Check sheet for the modelled part. Datum: model origin and axes. Units: mm. A direction names the side the tool comes from. Round coordinates to 2 decimals unless told otherwise and drop trailing zeros. Write each loop counter-clockwise with the first axis right and the second up, starting at its lowest first coordinate (ties: lowest second). Pieces come first, ordered by that corner, then holes. Notation, with made-up numbers: (-23.5, -34.5) -> (6.5, -34.5) arc R28 cw to (6.5, -13.5) -> close; hole circle Ø1 at (63.25, 37.25). An arc over 180 degrees is marked (long way). Write item = value, one per line.
from build123d import *

# Parameters (mm, degrees)
F1_DEPTH = 30
F3_DEPTH = 12
F5_D     = 16


with BuildPart() as f1:
    # F0 (on Right) → F1 (new body)
    with BuildSketch(Plane.YZ):
        Polygon((-20, -22.5), (20, -22.5), (110, -22.5), (110, -10.5), (20, -10.5), (20, 22.5), (-20, 22.5), align=None)
    extrude(amount=F1_DEPTH)

    # F2 (on face) → F3 (cut)
    with BuildSketch(Plane.XY.offset(-10.5)):
        with BuildLine():
            ThreePointArc((10.5, 103), (7, 106.5), (3.5, 103))
            Line((3.5, 103), (3.5, 83))
            ThreePointArc((3.5, 83), (7, 79.5), (10.5, 83))
            Line((10.5, 83), (10.5, 103))
        make_face()
        with BuildLine():
            Line((26.5, 82.575567), (26.5, 103))
            ThreePointArc((26.5, 103), (23, 106.5), (19.5, 103))
            Line((19.5, 103), (19.5, 82.575567))
            ThreePointArc((19.5, 82.575567), (23, 79.075567), (26.5, 82.575567))
        make_face()
    extrude(amount=-F3_DEPTH, mode=Mode.SUBTRACT)

    # F5 (through all)
    with Locations(Plane.XY.offset(22.5)):
        with Locations((15, -8)):
            Hole(F5_D / 2)


solid = f1.part
(1) Access from +Z, -Z, +X, -X, +Y, -Y to the whole of each face (thin tool, end or side, straight path). Record for faces 4 (the flat face through (15, 110, -17)), 5 (the flat face through (15, 20, 6)), 6 (the flat face through (10.5, 93, -16)).
Worked answers:
face_4 = +Z, -Z, +X, -X, +Y
face_5 = +Z, +X, -X, +Y
face_6 = +Z, -Z
(2) Go/stop test with flat-tipped pins: P1, Ø12, axis at y = 91, z = -14.5, coming from the -X side; P2, Ø3, axis at x = 19.5, y = 29, coming from the +Z side; P3, Ø15, axis at x = 20.5, z = 10, coming from the +Y side. Record where each tip stops, or that it passes through.
Worked answers:
P1 = 0
P2 = -10.5
P3 = 20
(3) Sectioned sample at A-A on y = -8. Enter the section's corners in (x, z), then the cut area to 3 significant figures.
Worked answers:
outline = (0, -22.5) -> (7, -22.5) -> (7, 22.5) -> (0, 22.5) -> close; (23, -22.5) -> (30, -22.5) -> (30, 22.5) -> (23, 22.5) -> close
area = 630 mm²
(4) Sectioned sample at B-B on x = 15. Enter the section's corners in (y, z).
Worked answers:
outline = (-20, -22.5) -> (-16, -22.5) -> (-16, 22.5) -> (-20, 22.5) -> close; (0, -22.5) -> (110, -22.5) -> (110, -10.5) -> (20, -10.5) -> (20, 22.5) -> (0, 22.5) -> close
(5) Release check for a two-part mould opening along X. For faces 1 (the flat face through (30, 15, -5)), 2 (the flat face through (19.5, 93, -16)), 3 (the flat face through (0, 15, -5)) record: pulls with the +X half, pulls with the -X half, needs draft (parallel to the pull), parting line crosses it, or undercut.
Worked answers:
face_1 = pulls with the +X half
face_2 = undercut
face_3 = pulls with the -X half
(6) Material ranges on L1, parallel to X at y = 86, z = -20; L2, parallel to Y at x = 15, z = -7.5; L3, parallel to Z at x = 2, y = 104, recorded low to high. Write a range as [from, to].
Worked answers:
L1 = [0, 3.5], [10.5, 19.5], [26.5, 30]
L2 = [-20, -16], [0, 20]
L3 = [-22.5, -10.5]
(7) Sectioned sample at D-D on z = -2.5. Enter the section's corners in (x, y), then the cut area to 3 significant figures.
Worked answers:
outline = (0, -20) -> (30, -20) -> (30, 20) -> (0, 20) -> close; hole circle Ø16 at (15, -8)
area = 999 mm²
(8) Sectioned sample at C-C on y = 88. Enter the section's corners in (x, z).
Worked answers:
outline = (0, -22.5) -> (3.5, -22.5) -> (3.5, -10.5) -> (0, -10.5) -> close; (10.5, -22.5) -> (19.5, -22.5) -> (19.5, -10.5) -> (10.5, -10.5) -> close; (26.5, -22.5) -> (30, -22.5) -> (30, -10.5) -> (26.5, -10.5) -> close
